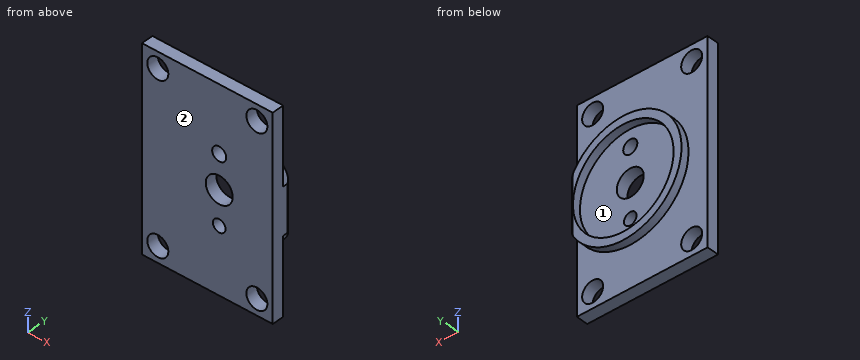
```python
from build123d import *

# Parameters (mm, degrees)
SKETCH1_W           = 25
SKETCH1_H           = 50
SKETCH1_R           = 3.4
BOSS_EXTRUDE1_DEPTH = 3
SKETCH2_W           = 50
SKETCH2_H           = 3
BOSS_EXTRUDE2_DEPTH = 8
SKETCH3_W           = 8
SKETCH3_H           = 50
BOSS_EXTRUDE3_DEPTH = 42
SKETCH4_R           = 2.65
CUT_EXTRUDE1_DEPTH  = 3.3
SKETCH5_R           = 5.802370205
CUT_EXTRUDE2_DEPTH  = 9
FILLET2_R           = 1
SKETCH6_R           = 12.7
BOSS_EXTRUDE4_DEPTH = 2
FILLET4_R           = 1
SKETCH8_R           = 1.589780168
SKETCH8_R_2         = 1.777428262
CUT_EXTRUDE3_DEPTH  = 10
SKETCH9_W           = 8
SKETCH9_H           = 42
CUT_EXTRUDE4_DEPTH  = 68.79439129


with BuildPart() as part:
    # Sketch1 → Boss-Extrude1 (new body)
    with BuildSketch(Plane(origin=(0, 0, 0), x_dir=(1, 0, 0), z_dir=(0, 1, 0))):
        with Locations((2.276951673, 11.384758364)):
            Rectangle(SKETCH1_W, SKETCH1_H)
        with Locations(Location((1.276951673, 11.384758364, 0), (0, 0, 270))):
            Circle(SKETCH1_R, mode=Mode.SUBTRACT)
    extrude(amount=BOSS_EXTRUDE1_DEPTH)

    # Sketch2 → Boss-Extrude2 (add)
    with BuildSketch(Plane.ZY.offset(10.223048327)):
        with Locations((-11.384758364, 1.5)):
            Rectangle(SKETCH2_W, SKETCH2_H)
    extrude(amount=BOSS_EXTRUDE2_DEPTH)

    # Sketch3 → Boss-Extrude3 (add)
    with BuildSketch(Plane.XZ):
        with Locations((-14.223048327, -11.384758364)):
            Rectangle(SKETCH3_W, SKETCH3_H)
    extrude(amount=BOSS_EXTRUDE3_DEPTH)

    # Sketch4 → Cut-Extrude1 (cut)
    with BuildSketch(Plane(origin=(0, 3, 0), x_dir=(1, 0, 0), z_dir=(0, 1, 0))):
        with Locations(Location((-14.223048327, 32.384758364, 0), (0, 0, 270))):
            Circle(SKETCH4_R)
        with Locations(Location((-14.223048327, -9.615241636, 0), (0, 0, 270))):
            Circle(SKETCH4_R)
    cut_extrude1 = extrude(amount=-CUT_EXTRUDE1_DEPTH, mode=Mode.SUBTRACT)

    # Mirror1: Cut-Extrude1 across plane
    add(cut_extrude1.mirror(Plane.ZX.offset(-19.5)), mode=Mode.SUBTRACT)

    # Sketch5 → Cut-Extrude2 (cut)
    with BuildSketch(Plane.ZY.offset(18.223048327)):
        with Locations((-11.836279124, -21)):
            Circle(SKETCH5_R)
    extrude(amount=-CUT_EXTRUDE2_DEPTH, mode=Mode.SUBTRACT)

    # Fillet2
    fillet2_edges = [part.edges().sort_by_distance(p)[0] for p in [
        (-10.223048327, -21, -17.638649329),
    ]]
    fillet(fillet2_edges, radius=FILLET2_R)

    # Mirror2: Cut-Extrude1 across plane
    add(cut_extrude1.mirror(Plane.ZY.offset(1.723048327)), mode=Mode.SUBTRACT)

    # Sketch6 → Boss-Extrude4 (add)
    with BuildSketch(Plane(origin=(0, 3, 0), x_dir=(1, 0, 0), z_dir=(0, 1, 0))):
        with BuildLine():
            Line((14.776951673, 5.567542535), (14.776951673, 17.201974193))
            ThreePointArc((14.776951673, 17.201974193), (-13.423048327, 11.384758364), (14.776951673, 5.567542535))
        make_face()
        with Locations(Location((1.276951673, 11.384758364, 0), (0, 0, 270))):
            Circle(SKETCH6_R, mode=Mode.SUBTRACT)
    extrude(amount=BOSS_EXTRUDE4_DEPTH)

    # Fillet4
    # the kernel refuses this fillet: 1 mm, written as the material it takes off along each edge
    with BuildSketch(Plane(origin=(14.776951673, 5, -3.067542535), x_dir=(0, -1, 0), z_dir=(0, 0, -1))) as fillet4_piece_1:
        with BuildLine():
            CenterArc((FILLET4_R, FILLET4_R), FILLET4_R, 180, 90)
            Line((0, FILLET4_R), (0, 0))
            Line((0, 0), (FILLET4_R, 0))
        make_face()
    extrude(amount=16.634431658, mode=Mode.SUBTRACT)

    # Sketch8 → Cut-Extrude3 (cut)
    with BuildSketch(Plane(origin=(0, 3, 0), x_dir=(1, 0, 0), z_dir=(0, 1, 0))):
        with Locations(Location((1.276951673, 19.884758364, 0), (0, 0, 270))):
            Circle(SKETCH8_R)
        with Locations(Location((1.276951673, 2.884758364, 0), (0, 0, 270))):
            Circle(SKETCH8_R_2)
    extrude(amount=-CUT_EXTRUDE3_DEPTH, mode=Mode.SUBTRACT)

    # Sketch9 → Cut-Extrude4 (cut, through all)
    with BuildSketch(Plane.XY.offset(13.615241636)):
        with Locations((-14.223048327, -21)):
            Rectangle(SKETCH9_W, SKETCH9_H)
    extrude(amount=-CUT_EXTRUDE4_DEPTH, mode=Mode.SUBTRACT)


solid = part.part
```
Geometry check sheet. Reference: the model listing, model coordinates, mm. Face numbers are marked on the shaded views. Give positions to 0.01 mm unless a question says otherwise; leave off trailing zeros. Loops run counter-clockwise (first coordinate to the right, second up) from the corner with the lowest first, then second, coordinate; pieces in that order, holes last. Notation, with made-up numbers: M -13,6 L 6,6 A11 cw 6,18 Z; hole C -35,-25.5 d4. An arc over 180 degrees is marked long. Answer as CSV lines item,"result".
Item 1: Release check for a two-part mould opening along Z. For the marked faces 1 and 2 record: pulls with the +Z half, pulls with the -Z half, needs draft (parallel to the pull), parting line crosses it, or undercut.
Values:
face 1,"undercut"
face 2,"needs draft"
Item 2: Cross-section at B-B on x = 2. Record the cut outline in (y, z), and give its area (3 significant figures).
Values:
outline,"M 0,-36.38 L 3,-36.38 L 3,-26.07 L 5,-26.07 L 5,-24.06 L 3,-24.06 L 3,-21.3 L 0,-21.3 Z; M 0,-18.47 L 3,-18.47 L 3,-14.71 L 0,-14.71 Z; M 0,-8.06 L 3,-8.06 L 3,-4.51 L 0,-4.51 Z; M 0,-1.26 L 3,-1.26 L 3,1.29 L 5,1.29 L 5,3.3 L 3,3.3 L 3,13.62 L 0,13.62 Z"
area,"120 mm²"
Item 3: Cross-section at D-D on x = -4. Record the cut outline in (y, z).
Values:
outline,"M 0,-36.38 L 3,-36.38 L 3,-25.1 L 5,-25.1 L 5,-22.94 L 3,-22.94 L 3,0.17 L 5,0.17 L 5,2.34 L 3,2.34 L 3,13.62 L 0,13.62 Z"
Item 4: Material ranges on line 1 (Z direction, x = -14, y = 1.55); line 2 (Z direction, x = 1.5, y = 2.2); line 3 (X direction, y = 0.35, z = -20), recorded low to high.
Values:
line 1,"z = -36.38 to -35.03, -29.74 to 6.97, 12.26 to 13.62"
line 2,"z = -36.38 to -21.46, -18.31 to -14.78, -7.99 to -4.65, -1.12 to 13.62"
line 3,"x = -18.22 to -0.31, 2.86 to 14.78"
Item 5: Cross-section at A-A on x = 11.5. Record the cut outline in (y, z).
Values:
outline,"M 0,-36.38 L 3,-36.38 L 3,-34.93 L 0,-34.93 Z; M 0,-29.84 L 3,-29.84 L 3,-21.95 L 5,-21.95 L 5,-18.92 L 3,-18.92 L 3,-3.85 L 5,-3.85 L 5,-0.82 L 3,-0.82 L 3,7.07 L 0,7.07 Z; M 0,12.16 L 3,12.16 L 3,13.62 L 0,13.62 Z"
Item 6: Cross-section at C-C on z = -25.5. Record the cut outline in (x, y), and give its area (3 significant figures).
Values:
outline,"M -18.22,0 L 14.78,0 L 14.78,3 L 5.38,3 L 5.38,5 L -2.83,5 L -2.83,3 L -18.22,3 Z"
area,"115 mm²"
